from build123d import *

# Parameters (mm, degrees)
SKETCH3_R           = 0.635
BOSS_EXTRUDE1_DEPTH = 1.27


with BuildPart() as part:
    # Sketch2 → Revolve1 (revolve)
    with BuildSketch(Plane.XY):
        Polygon((0, 0), (0, 2.54), (26.162, 2.54), (26.162, 0), (25.146, 0), (25.146, -1.27), (24.13, -1.27), (24.13, 0), align=None)
    revolve(axis=Axis((0, -1000, 0), (0, 1, 0)))

    # Sketch3 → Boss-Extrude1 (add, symmetric)
    with BuildSketch(Plane.XY):
        with BuildLine():
            Line((-25.4, 1.651), (-25.4, 0))
            Line((-25.4, 0), (-26.924, 0))
            ThreePointArc((-26.924, 0), (-27.7495, 0.8255), (-26.924, 1.651))
            Line((-26.924, 1.651), (-25.4, 1.651))
        make_face()
        with Locations((-26.924, 0.8255)):
            Circle(SKETCH3_R, mode=Mode.SUBTRACT)
    extrude(amount=BOSS_EXTRUDE1_DEPTH, both=True)


solid = part.part
Source: CAD feature listing. Evaluate the final solid. Frame: model axes, mm. A direction names the side the tool comes from. Coordinates: 2 decimals unless noted, no trailing zeros. Loops run counter-clockwise (first coordinate to the right, second up) from the corner with the lowest first, then second, coordinate; pieces in that order, holes last. Notation, with made-up numbers: M 23.5,9 L 56.5,9 A23 cw 56.5,45 Z; hole C 62,-16.5 d7. An arc over 180 degrees is marked long. Answer in a Markdown table with one row per item.
Q1. Ray query, probe 1 along Z at (x, y) = (-0.5, -0.4); probe 2 along X at (y, z) = (-0.4, 0); probe 3 along X at (y, z) = (2.3, 0). Return the intervals inside material, ascending. Write a range as from..to.
Answers below:
| item | result |
|---|---|
| probe 1 | z = -25.14..-24.12, 24.12..25.14 |
| probe 2 | x = -25.15..-24.13, 24.13..25.15 |
| probe 3 | x = -26.16..26.16 |
Q2. Section B-B on y = -0.65. Return the cut outline in (x, z), plus the area to 3 significant figures.
Answers below:
| item | result |
|---|---|
| outline | C 0,0 d50.29; hole C 0,0 d48.26 |
| area | 157 mm^2 |
Q3. Section C-C on z = 4.5. Return the cut outline in (x, y).
Answers below:
| item | result |
|---|---|
| outline | M -25.77,0 L -24.74,0 L -24.74,-1.27 L -23.71,-1.27 L -23.71,0 L 23.71,0 L 23.71,-1.27 L 24.74,-1.27 L 24.74,0 L 25.77,0 L 25.77,2.54 L -25.77,2.54 Z |
Q4. Draft query along X for faces 1 (the flat face through (0, 2.54, 0)), 2 (the cylindrical face through (24.954, 1.252, -7.858)), 3 (the cylindrical face through (23.016, -0.626, -7.248)). Return one class per face: pulls with the +X half, pulls with the -X half, needs draft (parallel to the pull), parting line crosses it, or undercut.
Answers below:
| item | result |
|---|---|
| face 1 | needs draft |
| face 2 | parting line crosses it |
| face 3 | undercut |
Q5. First-contact query: pin 1 (0.8 mm diameter, centred on x = -26.92, y = 0.83, fed in from -Z); pin 2 (1.5 mm diameter, centred on x = -15, y = -0.5, fed in from -Z); pin 3 (1 mm diameter, centred on x = -17, y = 0, fed in from +Z); pin 4 (2 mm diameter, centred on x = -10.5, y = 0.5, fed in from -Z). Flat tips, straight axial feed; report the tip coordinate or a pass-through.
Answers below:
| item | result |
|---|---|
| pin 1 | passes through |
| pin 2 | stops at z = -21.82 |
| pin 3 | stops at z = 20.3 |
| pin 4 | stops at z = -24.38 |
Q6. Set-up query: faces 4 (the flat face through (-9.4, -1.27, -22.5)), 5 (the flat face through (0, 0, 0)). Return all of +Z, -Z, +X, -X, +Y, -Y with unobstructed straight access to the full face (end or side cutting, diameter ignored); none if empty.
Answers below:
| item | result |
|---|---|
| face 4 | +Z, -Z, +X, -X, -Y |
| face 5 | -Y |
Q7. Section A-A on x = 0. Return the cut outline in (y, z), plus the area to 3 significant figures.
Answers below:
| item | result |
|---|---|
| outline | M -1.27,-25.15 L 0,-25.15 L 0,-26.16 L 2.54,-26.16 L 2.54,26.16 L 0,26.16 L 0,25.15 L -1.27,25.15 L -1.27,24.13 L 0,24.13 L 0,-24.13 L -1.27,-24.13 Z |
| area | 135 mm^2 |
